```python
from build123d import *

# Parameters (mm, degrees)
F1_DEPTH = 25.4


with BuildPart() as f1:
    # F0 (on Front) → F1 (new body)
    with BuildSketch(Plane.XZ):
        with BuildLine():
            ThreePointArc((-72.749855, 63.382049), (-72.700367, 63.959206), (-72.683854, 64.538244))
            ThreePointArc((-72.683854, 64.538244), (-83.422892, 74.681731), (-92.937852, 63.382049))
            ThreePointArc((-92.937852, 63.382049), (-82.843854, 54.378244), (-72.749855, 63.382049))
        make_face()
        with BuildLine():
            ThreePointArc((-72.749855, 63.382049), (-82.843854, 54.378244), (-92.937852, 63.382049))
            Line((-92.937852, 63.382049), (-92.937852, 12.293785))
            Line((-92.937852, 12.293785), (-72.749855, 12.293785))
            Line((-72.749855, 12.293785), (-72.749855, 63.382049))
        make_face()
        Polygon((-72.749855, 12.293785), (-92.937852, 12.293785), (-113.261852, 12.293785), (-133.44985, 12.293785), (-153.85941, 12.293785), (-174.047408, 12.293785), (-174.047408, -38.506215), (-173.53265, -48.624064), (-144.623931, -48.624064), (130.419544, -48.624064), (129.97048, -37.800175), (129.97048, 12.293785), (109.782483, 12.293785), (89.372952, 12.293785), (69.184954, 12.293785), (48.775379, 12.293785), (28.587381, 12.293785), (8.312916, 12.293785), (-11.875082, 12.293785), (-32.126242, 12.293785), (-52.314239, 12.293785), align=None)
        with BuildLine():
            Line((-133.44985, 12.293785), (-113.261852, 12.293785))
            Line((-113.261852, 12.293785), (-113.261852, 63.093788))
            ThreePointArc((-113.261852, 63.093788), (-123.355851, 54.089983), (-133.44985, 63.093788))
            Line((-133.44985, 63.093788), (-133.44985, 12.293785))
        make_face()
        with BuildLine():
            Line((-52.314239, 63.374581), (-52.314239, 12.293785))
            Line((-52.314239, 12.293785), (-32.126242, 12.293785))
            Line((-32.126242, 12.293785), (-32.126242, 63.374581))
            ThreePointArc((-32.126242, 63.374581), (-42.220241, 54.370776), (-52.314239, 63.374581))
        make_face()
        with BuildLine():
            ThreePointArc((-133.44985, 63.093788), (-123.355851, 54.089983), (-113.261852, 63.093788))
            ThreePointArc((-113.261852, 63.093788), (-113.212364, 63.670944), (-113.195851, 64.249983))
            ThreePointArc((-113.195851, 64.249983), (-123.934889, 74.393469), (-133.44985, 63.093788))
        make_face()
        with BuildLine():
            ThreePointArc((-32.060241, 64.530776), (-42.799279, 74.674262), (-52.314239, 63.374581))
            ThreePointArc((-52.314239, 63.374581), (-42.220241, 54.370776), (-32.126242, 63.374581))
            ThreePointArc((-32.126242, 63.374581), (-32.076754, 63.951737), (-32.060241, 64.530776))
        make_face()
        with BuildLine():
            Line((-174.047408, 12.293785), (-153.85941, 12.293785))
            Line((-153.85941, 12.293785), (-153.85941, 63.093785))
            ThreePointArc((-153.85941, 63.093785), (-163.953409, 54.08998), (-174.047408, 63.093785))
            Line((-174.047408, 63.093785), (-174.047408, 12.293785))
        make_face()
        with BuildLine():
            Line((-11.875082, 63.37458), (-11.875082, 12.293785))
            Line((-11.875082, 12.293785), (8.312916, 12.293785))
            Line((8.312916, 12.293785), (8.312916, 63.37458))
            ThreePointArc((8.312916, 63.37458), (-1.781083, 54.370775), (-11.875082, 63.37458))
        make_face()
        with BuildLine():
            ThreePointArc((-174.047408, 63.093785), (-163.953409, 54.08998), (-153.85941, 63.093785))
            ThreePointArc((-153.85941, 63.093785), (-153.809922, 63.670941), (-153.793409, 64.24998))
            ThreePointArc((-153.793409, 64.24998), (-164.532447, 74.393466), (-174.047408, 63.093785))
        make_face()
        with BuildLine():
            ThreePointArc((8.378917, 64.530775), (-2.360122, 74.674261), (-11.875082, 63.37458))
            ThreePointArc((-11.875082, 63.37458), (-1.781083, 54.370775), (8.312916, 63.37458))
            ThreePointArc((8.312916, 63.37458), (8.362403, 63.951736), (8.378917, 64.530775))
        make_face()
        with BuildLine():
            Line((28.587381, 63.446807), (28.587381, 12.293785))
            Line((28.587381, 12.293785), (48.775379, 12.293785))
            Line((48.775379, 12.293785), (48.775379, 63.446807))
            ThreePointArc((48.775379, 63.446807), (38.68138, 54.443002), (28.587381, 63.446807))
        make_face()
        with BuildLine():
            ThreePointArc((48.84138, 64.603002), (38.102342, 74.746488), (28.587381, 63.446807))
            ThreePointArc((28.587381, 63.446807), (38.68138, 54.443002), (48.775379, 63.446807))
            ThreePointArc((48.775379, 63.446807), (48.824867, 64.023963), (48.84138, 64.603002))
        make_face()
        with BuildLine():
            Line((69.184954, 63.446804), (69.184954, 12.293785))
            Line((69.184954, 12.293785), (89.372952, 12.293785))
            Line((89.372952, 12.293785), (89.372952, 63.446804))
            ThreePointArc((89.372952, 63.446804), (79.278953, 54.442999), (69.184954, 63.446804))
        make_face()
        with BuildLine():
            ThreePointArc((89.438953, 64.602999), (78.699915, 74.746485), (69.184954, 63.446804))
            ThreePointArc((69.184954, 63.446804), (79.278953, 54.442999), (89.372952, 63.446804))
            ThreePointArc((89.372952, 63.446804), (89.42244, 64.023961), (89.438953, 64.602999))
        make_face()
        with BuildLine():
            Line((109.782483, 63.799825), (109.782483, 12.293785))
            Line((109.782483, 12.293785), (129.97048, 12.293785))
            Line((129.97048, 12.293785), (129.97048, 63.799825))
            ThreePointArc((129.97048, 63.799825), (119.876481, 54.79602), (109.782483, 63.799825))
        make_face()
        with BuildLine():
            ThreePointArc((130.036481, 64.95602), (119.297443, 75.099506), (109.782483, 63.799825))
            ThreePointArc((109.782483, 63.799825), (119.876481, 54.79602), (129.97048, 63.799825))
            ThreePointArc((129.97048, 63.799825), (130.019968, 64.376981), (130.036481, 64.95602))
        make_face()
    extrude(amount=F1_DEPTH)


solid = f1.part
```
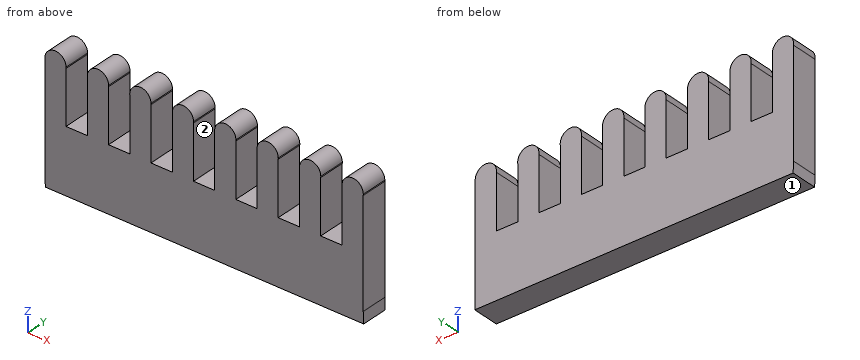
Geometry check sheet. Reference: the model listing, model coordinates, mm. Face numbers are marked on the shaded views. Coordinates: 2 decimals unless noted, no trailing zeros. Loops run counter-clockwise (first coordinate to the right, second up) from the corner with the lowest first, then second, coordinate; pieces in that order, holes last.
Item 1: Sectioned sample at A-A, the plane z = 29. Count the separate pieces of the cut face and the enclosed holes in it, then the cut area to 3 significant figures.
Item 2: Go/stop test with flat-tipped pins: pin 1 Ø7.5 at (y, z) = (-6.5, 33.5) entering from -X; pin 2 Ø12.5 at (y, z) = (-13.5, 43) entering from +X; pin 3 Ø12 at (y, z) = (-14.5, 57.5) entering from -X. Record where each tip stops, or that it passes through.
Item 3: Sectioned sample at B-B, the plane x = 60.5. Record the boundary of the cut face in (y, z), then the cut area to 3 significant figures.
Item 4: Release check for a two-part mould opening along X. For the marked faces 1 and 2 record: released by +X, released by -X, zero draft, split by the parting line, or undercut.
Item 5: Thickness scan on line 1 (Z direction, x = -14, y = -22); line 2 (X direction, y = -16.25, z = -13.5); line 3 (Z direction, x = -122.5, y = -3.75). Record the ranges inside material, lowest first.
Check result:
1. separate pieces: 8
1. enclosed holes: 0
1. area: 4,100 mm2
2. pin 1: stops at x = -174.05
2. pin 2: stops at x = 129.97
2. pin 3: stops at x = -174.09
3. outline: (-25.4, -48.62) - (0, -48.62) - (0, 12.29) - (-25.4, 12.29) - close
3. area: 1,550 mm2
4. face 1: zero draft
4. face 2: undercut
5. line 1: z = -48.62 to 12.29
5. line 2: x = -174.05 to 129.97
5. line 3: z = -48.62 to 74.37
